from build123d import *

# Parameters (mm, degrees)
EXTRUDE_1_DEPTH = 5
SKETCH_3_R      = 2.5
EXTRUDE_2_DEPTH = 5


with BuildPart() as part:
    # 草图2 → 凸台-拉伸1 (new body)
    with BuildSketch(Plane(origin=(0, 0, 0), x_dir=(1, 0, 0), z_dir=(0, 1, 0))):
        Polygon((-120, -150), (-120, -135), (120, -135), (120, -150), (150, -150), (150, -120), (135, -120), (135, 120), (150, 120), (150, 150), (120, 150), (120, 135), (-120, 135), (-120, 150), (-150, 150), (-150, 120), (-135, 120), (-135, -120), (-150, -120), (-150, -150), align=None)
    extrude(amount=EXTRUDE_1_DEPTH)

    # 草图3 → 凸台-拉伸2 (add)
    with BuildSketch(Plane(origin=(0, 0, 0), x_dir=(1, 0, 0), z_dir=(0, 1, 0))):
        with Locations(Location((-88.388347648, 88.388347648, 0), (0, 0, 270))):
            Circle(SKETCH_3_R)
        with Locations(Location((88.388347648, 88.388347648, 0), (0, 0, 270))):
            Circle(SKETCH_3_R)
        with Locations(Location((-88.388347648, -88.388347648, 0), (0, 0, 270))):
            Circle(SKETCH_3_R)
        with Locations(Location((88.388347648, -88.388347648, 0), (0, 0, 270))):
            Circle(SKETCH_3_R)
    extrude(amount=-EXTRUDE_2_DEPTH)


solid = part.part
Geometry: final body of the model. Coordinates: model frame, mm. Give positions to 0.01 mm unless a question says otherwise; leave off trailing zeros. Write each loop counter-clockwise with the first axis right and the second up, starting at its lowest first coordinate (ties: lowest second). Pieces come first, ordered by that corner, then holes. Notation, with made-up numbers: (-23, 86) -> (-5, 86) arc R14 cw to (-5, 110) -> close; hole circle Ø10 at (51.5, 24.25). An arc over 180 degrees is marked (long way). Answer in a Markdown table with one row per item.
(1) Pin query (flat end, axial travel): pin 1 (2 mm diameter, centred on y = -2, z = -24.5, fed in from +X); pin 2 (4 mm diameter, centred on x = 26.5, y = 3.5, fed in from -Z); pin 3 (1.5 mm diameter, centred on y = 1.5, z = -26.5, fed in from -X); pin 4 (8 mm diameter, centred on x = 78, z = 109, fed in from -Y). Return the tip coordinate at first contact, or that it passes through.
Answers below:
| item | result |
|---|---|
| pin 1 | through |
| pin 2 | z = -135 |
| pin 3 | x = -135 |
| pin 4 | y = 0 |
(2) Section query C-C on z = 39.5. Return loops of the section in (x, y).
Answers below:
| item | result |
|---|---|
| outline | (-135, 0) -> (135, 0) -> (135, 5) -> (-135, 5) -> close |
(3) Section query B-B on x = -10.5. Return loops of the section in (y, z).
Answers below:
| item | result |
|---|---|
| outline | (0, -135) -> (5, -135) -> (5, 135) -> (0, 135) -> close |
(4) Section query A-A on y = 3.25. Return loops of the section in (x, z), then the cut area to 3 significant figures.
Answers below:
| item | result |
|---|---|
| outline | (-150, -150) -> (-120, -150) -> (-120, -135) -> (120, -135) -> (120, -150) -> (150, -150) -> (150, -120) -> (135, -120) -> (135, 120) -> (150, 120) -> (150, 150) -> (120, 150) -> (120, 135) -> (-120, 135) -> (-120, 150) -> (-150, 150) -> (-150, 120) -> (-135, 120) -> (-135, -120) -> (-150, -120) -> close |
| area | 75,600 mm^2 |
(5) Ray query, line 1 along Z through (x, y) = (138, 2.25); line 2 along Y through (x, z) = (104, 34.5); line 3 along X through (y, z) = (1.5, -112.5). Return the intervals inside material, ascending. Write a range as [from, to].
Answers below:
| item | result |
|---|---|
| line 1 | [-150, -120], [120, 150] |
| line 2 | [0, 5] |
| line 3 | [-135, 135] |
